Could you check a few things on this model? Use its own coordinates, in mm. Give positions to 0.01 mm unless a question says otherwise; leave off trailing zeros. Order: outer loops, then holes, each group sorted by start corner. A loop starts at its lowest first (then second) coordinate and runs counter-clockwise, first axis right, second up. Notation, with made-up numbers: M 28.5,55 L 45.5,55 A22 cw 45.5,72 Z; hole C -16.5,74.5 d6. An arc over 180 degrees is marked long. Use a Markdown table: item, result. Add a question column.
Item 1: Suppose I cut it at B-B on x = -0.5. Write out the boundary of the cut face in (y, z), plus the area to 3 significant figures.
Item 2: Suppose I cut it at C-C on y = 1.3. Count the separate pieces of the cut face and the enclosed holes in it, plus the area to 3 significant figures.
Item 3: I'm going to push a flat-ended pin straight in: pin 1 Ø3.5 at (x, z) = (28.51, 1.65) entering from +Y. Where does the tip first touch, or does it pass through?
Item 4: Suppose I cut it at A-A on z = 11.5. Write out the boundary of the cut face in (x, y), plus the area to 4 significant figures.
Item 5: If I drill on L1, parallel to X at y = 1, z = 14; L2, parallel to Z at x = -74, y = 2.25; L3, parallel to X at y = 0.8, z = -34, over which ranges is the centre line in solid material (lowest first)? Write a range as from..to.
Item 6: If we mould it in two halves opening along Z, with no side actions, what happens to faces 1 (the face through (-42, 1, -40.354)), 2 (the face through (-115.488, 1, 2)), 3 (the face through (27.012, 1, 12))? For each: released by +Z, released by -Z, zero draft, split by the parting line, or undercut.
from build123d import *

# Parameters (mm, degrees)
SKETCH1_W           = 149.499999434
SKETCH1_H           = 84
BOSS_EXTRUDE1_DEPTH = 3
SKETCH2_W           = 20
SKETCH2_H           = 3
SKETCH2_W_2         = 3
SKETCH2_H_2         = 10
CUT_EXTRUDE1_DEPTH  = 124.496635409
SKETCH3_R           = 1.6
CUT_EXTRUDE2_DEPTH  = 124.496635409
FILLET1_R           = 3


with BuildPart() as part:
    # Sketch1 → Boss-Extrude1 (new body)
    with BuildSketch(Plane(origin=(0, 0, 0), x_dir=(1, 0, 0), z_dir=(0, 1, 0))):
        with Locations((-40.737898115, -1.645897993)):
            Rectangle(SKETCH1_W, SKETCH1_H)
    extrude(amount=BOSS_EXTRUDE1_DEPTH)

    # Sketch2 → Cut-Extrude1 (cut, through all)
    with BuildSketch(Plane.XZ):
        with Locations((2.012101602, -34.854102007)):
            Rectangle(SKETCH2_W, SKETCH2_H)
        with Locations((-83.487897832, -34.854102007)):
            Rectangle(SKETCH2_W, SKETCH2_H)
        with Locations((-83.487897832, 38.145897993)):
            Rectangle(SKETCH2_W, SKETCH2_H)
        with Locations((2.012101602, 38.145897993)):
            Rectangle(SKETCH2_W, SKETCH2_H)
        with Locations((-109.987897832, 11.645897993)):
            Rectangle(SKETCH2_W_2, SKETCH2_H_2)
        with Locations((-109.987897832, -8.354102007)):
            Rectangle(SKETCH2_W_2, SKETCH2_H_2)
        with Locations((28.512101602, 11.645897993)):
            Rectangle(SKETCH2_W_2, SKETCH2_H_2)
        with Locations((28.512101602, -8.354102007)):
            Rectangle(SKETCH2_W_2, SKETCH2_H_2)
    extrude(amount=-CUT_EXTRUDE1_DEPTH, mode=Mode.SUBTRACT)

    # Sketch3 → Cut-Extrude2 (cut, through all)
    with BuildSketch(Plane.XZ):
        with Locations(Location((28.512101602, 1.645897993, 0), (0, 0, 270))):
            Circle(SKETCH3_R)
        with Locations(Location((-109.987897832, 1.645897993, 0), (0, 0, 270))):
            Circle(SKETCH3_R)
    extrude(amount=-CUT_EXTRUDE2_DEPTH, mode=Mode.SUBTRACT)

    # Fillet1
    fillet1_edges = [part.edges().sort_by_distance(p)[0] for p in [
        (-115.487897832, 1.5, -40.354102007),
        (34.012101602, 1.5, -40.354102007),
        (34.012101602, 1.5, 43.645897993),
        (-115.487897832, 1.5, 43.645897993),
    ]]
    fillet(fillet1_edges, radius=FILLET1_R)


solid = part.part
Findings below:
| question | item | result |
|---|---|---|
| 1 | outline | M 0,-40.35 L 3,-40.35 L 3,-36.35 L 0,-36.35 Z; M 0,-33.35 L 3,-33.35 L 3,36.65 L 0,36.65 Z; M 0,39.65 L 3,39.65 L 3,43.65 L 0,43.65 Z |
| 1 | area | 234 mm^2 |
| 2 | separate pieces | 1 |
| 2 | enclosed holes | 10 |
| 2 | area | 12,200 mm^2 |
| 3 | pin 1 | stops at y = 3 |
| 4 | outline | M -115.49,0 L -111.49,0 L -111.49,3 L -115.49,3 Z; M -108.49,0 L 27.01,0 L 27.01,3 L -108.49,3 Z; M 30.01,0 L 34.01,0 L 34.01,3 L 30.01,3 Z |
| 4 | area | 430.5 mm^2 |
| 5 | L1 | x = -115.49..-111.49, -108.49..27.01, 30.01..34.01 |
| 5 | L2 | z = -40.35..-36.35, -33.35..36.65, 39.65..43.65 |
| 5 | L3 | x = -115.49..-93.49, -73.49..-7.99, 12.01..34.01 |
| 6 | face 1 | released by -Z |
| 6 | face 2 | zero draft |
| 6 | face 3 | undercut |
